from build123d import *

# Parameters (mm, degrees)
F0_R           = 1.016
F0_W           = 20.32
F0_H           = 40.64
F2_DEPTH       = 17.526
F3_DEPTH       = 63.5
F4_R           = 3.81
F5_DEPTH       = 6.35
F7_D           = 2.032
F7_CSINK_D     = 3.175
F7_CSINK_ANGLE = 82
F8_SIZE        = 0.254


with BuildPart() as f2:
    # F0 (on Top) → F2 (new body, through all)
    with BuildSketch(Plane.XY):
        with BuildLine():
            Line((15.24, 40.64), (-15.24, 40.64))
            Line((-15.24, 40.64), (-15.24, -13.97))
            Line((-15.24, -13.97), (-7.698966, -27.031454))
            ThreePointArc((-7.698966, -27.031454), (0, -31.476454), (7.698966, -27.031454))
            Line((7.698966, -27.031454), (15.24, -13.97))
            Line((15.24, -13.97), (15.24, 40.64))
        make_face()
        with Locations((-5.4991, -13.97)):
            Circle(F0_R, mode=Mode.SUBTRACT)
        with Locations((5.4991, -13.97)):
            Circle(F0_R, mode=Mode.SUBTRACT)
        with Locations((-5.4991, 34.036)):
            Circle(F0_R, mode=Mode.SUBTRACT)
        with Locations((0, 10.16)):
            Rectangle(F0_W, F0_H, mode=Mode.SUBTRACT)
        with Locations((5.4991, 34.036)):
            Circle(F0_R, mode=Mode.SUBTRACT)
    extrude(amount=-F2_DEPTH)

    # F1 (on Right) → F3 (intersect, symmetric)
    with BuildSketch(Plane.YZ):
        Polygon((-16.160291, 0), (-31.476454, 0), (-31.476454, -5.0606), (-21.016742, -17.526), (40.64, -17.526), (40.64, -11.176), (-9.766352, -11.176), (-16.160291, -3.556), align=None)
    extrude(amount=F3_DEPTH, both=True, mode=Mode.INTERSECT)

    # F4 (on face) → F5 (join)
    with BuildSketch(Plane.XY):
        with Locations((0, -22.86)):
            Circle(F4_R)
    extrude(amount=F5_DEPTH)

    # F7 (through all)
    with Locations(Plane.XY.offset(6.35)):
        with Locations((0, -22.86)):
            CounterSinkHole(F7_D / 2, F7_CSINK_D / 2, counter_sink_angle=F7_CSINK_ANGLE)

    # F8
    f8_edges = [f2.edges().sort_by_distance(p)[0] for p in [
        (-3.81, -22.86, 6.35),
    ]]
    chamfer(f8_edges, length=F8_SIZE)


solid = f2.part
Source: CAD feature listing. Evaluate the final solid. Frame: model axes, mm. A direction names the side the tool comes from. Round coordinates to 2 decimals unless told otherwise and drop trailing zeros. Loops run counter-clockwise (first coordinate to the right, second up) from the corner with the lowest first, then second, coordinate; pieces in that order, holes last. Notation, with made-up numbers: (80.5, 67.5) -> (86.5, 67.5) arc R37 cw to (86.5, 104.5) -> close; hole circle Ø5 at (57.5, -5). An arc over 180 degrees is marked (long way). Answer as a JSON object with one key per item and string values. Group by question number.
Q1. Section query C-C (x = 0). Output: boundary loops of the cut face in (y, z).
Q2. Section query A-A (y = -6.5). Output: boundary loops of the cut face in (x, z).
Q3. Section query B-B (z = -7.5). Output: boundary loops of the cut face in (x, y).
Q4. Ray query, line 1 (X direction, y = -13.97, z = -11); line 2 (Y direction, x = 0, z = -0.75); line 3 (X direction, y = 4, z = -13.25). Return the intervals inside material, ascending. Write a range as from..to.
Q5. Mould query, pull axis Y, two halves, no side actions, for faces 5 (the flat face through (0.16, -25.16, -12.59)), 6 (the cylindrical face through (-5.631, 35.043, -14.307)), 7 (the flat face through (2, -24, 6.35)). Classes: pulls with the +Y half, pulls with the -Y half, needs draft (parallel to the pull), parting line crosses it, or undercut.
Q6. Access query for faces 1 (the flat face through (3, -20, 0)), 2 (the flat face through (10.16, 10, -14)), 3 (the flat face through (10.4, 21.4, -11.176)), 4 (the flat face through (15.24, 13, -14)). Directions: +Z, -Z, +X, -X, +Y, -Y. A direction counts if a zero-diameter tool reaches every point of the face in a straight line with its end or side. Return the directions, or none.
Q7. Contact query for flat-ended pins moving along their axis: P1, Ø4, axis at x = 0.5, z = -1, coming from the +Y side; P2, Ø1.9, axis at x = 3.5, z = -14, coming from the -Y side; P3, Ø5, axis at x = 4.5, y = -9.5, coming from the -Z side; P4, Ø12, axis at x = 11.5, y = 15.5, coming from the +Z side. Output: stop coordinate, or through.
Q8. Section query D-D (z = -13.75). Output: boundary loops of the cut face in (x, y), plus the area to 3 significant figures.
Completed:
{
 "1": {"outline": "(-31.48, -5.06) -> (-23.88, -14.12) -> (-23.88, 5.69) -> (-24.45, 6.35) -> (-26.42, 6.35) -> (-26.67, 6.1) -> (-26.67, 0) -> (-31.48, 0) -> close; (-21.84, -16.54) -> (-21.02, -17.53) -> (-10.16, -17.53) -> (-10.16, -10.71) -> (-16.16, -3.56) -> (-16.16, 0) -> (-19.05, 0) -> (-19.05, 6.1) -> (-19.3, 6.35) -> (-21.27, 6.35) -> (-21.84, 5.69) -> close; (30.48, -17.53) -> (40.64, -17.53) -> (40.64, -11.18) -> (30.48, -11.18) -> close"},
 "2": {"outline": "(-15.24, -17.53) -> (-10.16, -17.53) -> (-10.16, -11.18) -> (-15.24, -11.18) -> close; (10.16, -17.53) -> (15.24, -17.53) -> (15.24, -11.18) -> (10.16, -11.18) -> close"},
 "3": {"outline": "(-15.24, -13.97) -> (-7.7, -27.03) arc R8.89 ccw to (-5.67, -29.43) -> (5.67, -29.43) arc R8.89 ccw to (7.7, -27.03) -> (15.24, -13.97) -> (15.24, -12.85) -> (-15.24, -12.85) -> close; hole circle Ø2.03 at (-5.5, -13.97); hole circle Ø2.03 at (0, -22.86); hole circle Ø2.03 at (5.5, -13.97)"},
 "4": {"line 1": "-15.24..-6.52, -4.48..4.48, 6.52..15.24", "line 2": "-31.48..-23.88, -21.84..-16.16", "line 3": "-15.24..-10.16, 10.16..15.24"},
 "5": {"face 5": "pulls with the -Y half", "face 6": "undercut", "face 7": "needs draft"},
 "6": {"face 1": "+Z", "face 2": "+Z, -Z", "face 3": "+Z, +X, -X, +Y", "face 4": "+Z, -Z, +X, +Y, -Y"},
 "7": {"P1": "y = -16.16", "P2": "y = -24.77", "P3": "z = -17.53", "P4": "z = -11.18"},
 "8": {"outline": "(-15.24, -13.97) -> (-9.34, -24.19) -> (9.34, -24.19) -> (15.24, -13.97) -> (15.24, 40.64) -> (-15.24, 40.64) -> close; hole (-10.16, -10.16) -> (10.16, -10.16) -> (10.16, 30.48) -> (-10.16, 30.48) -> close; hole circle Ø2.03 at (-5.5, -13.97); hole circle Ø2.03 at (-5.5, 34.04); hole circle Ø2.03 at (0, -22.86); hole circle Ø2.03 at (5.5, -13.97); hole circle Ø2.03 at (5.5, 34.04)", "area": "1,070 mm²"}
}
